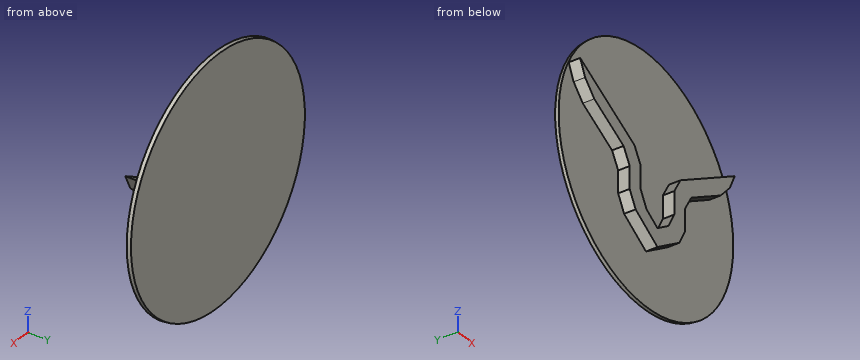
from build123d import *

# Parameters (mm, degrees)
PAD_DEPTH    = 20
SKETCH001_R  = 160.213684
PAD001_DEPTH = 5
PAD001_TAPER = -7
CHAMFER_SIZE = 13


with BuildPart() as part:
    # Sketch → Pad (new body)
    with BuildSketch(Plane.XZ):
        Polygon((0, -88.645294), (51.118267, -54.973317), (51.118267, 0), (127.669846, 44.197075), (142.406095, 75.799063), (31.118267, 11.547005), (31.118267, -44.19839), (0, -64.69622), (-31.118267, -44.19839), (-31.118267, 11.547005), (-142.406095, 75.799063), (-127.669846, 44.197075), (-51.118267, 0), (-51.118267, -54.973317), align=None)
    extrude(amount=PAD_DEPTH)

    # Sketch001 → Pad001 (join)
    with BuildSketch(Plane.XZ):
        with Locations((0, 2.38974)):
            Circle(SKETCH001_R)
    extrude(amount=PAD001_DEPTH, taper=PAD001_TAPER)

    # Chamfer
    chamfer_edges = [part.edges().sort_by_distance(p)[0] for p in [
        (31.118267, -12.5, 11.547005),
        (31.118267, -12.5, -44.19839),
        (-51.118267, -12.5, -54.973317),
        (-51.118267, -12.5, 0),
        (-127.669846, -12.5, 44.197075),
        (-31.118267, -12.5, 11.547005),
        (-31.118267, -12.5, -44.19839),
        (51.118267, -12.5, -54.973317),
        (51.118267, -12.5, 0),
        (127.669846, -12.5, 44.197075),
    ]]
    chamfer(chamfer_edges, length=CHAMFER_SIZE)


solid = part.part
For this review, take the finished solid that the model builds, in its own axes (mm). Round coordinates to 2 decimals unless told otherwise and drop trailing zeros. Write each loop counter-clockwise with the first axis right and the second up, starting at its lowest first coordinate (ties: lowest second). Pieces come first, ordered by that corner, then holes. Notation, with made-up numbers: M 36.25,43.25 L 64.25,43.25 A24 ccw 64.25,72.25 Z; hole C 47.5,76 d10. An arc over 180 degrees is marked long. Write item = value, one per line. Start each with the question number.
(1) We need section A-A (y = -11.5). Give the boundary of the cut face in (x, z), then the cut area to 3 significant figures.
(2) Clearance check with flat-ended pins moving along their axes: pin 1 Ø5 at (x, y) = (44, -4) entering from -Z; pin 2 Ø1.5 at (x, y) = (42.5, -9) entering from -Z; pin 3 Ø5 at (x, y) = (-39.5, -9.5) entering from +Z. State where each tip first meets the part, or that it passes through.
(3) For line 1 along Y through (x, z) = (15, 113.5); line 2 along X through (y, z) = (-12.25, 61); line 3 along X through (y, z) = (-10.75, -41), list the stretches that pass through material, from the lowest coordinate up.
Results found:
q1.outline = M -142.41,75.8 L -133.16,55.98 L -116.41,37.7 L -62.38,6.5 L -51.12,-13 L -51.12,-41.97 L -40.26,-62.12 L 0,-88.65 L 40.26,-62.12 L 51.12,-41.97 L 51.12,-13 L 62.38,6.5 L 116.41,37.7 L 133.16,55.98 L 142.41,75.8 L 42.38,18.05 L 31.12,-1.45 L 31.12,-31.2 L 20.26,-51.35 L 0,-64.7 L -20.26,-51.35 L -31.12,-31.2 L -31.12,-1.45 L -42.38,18.05 Z
q1.area = 8,420 mm²
q2.pin_1 = -152.94
q2.pin_2 = -59.36
q2.pin_3 = 17.39
q3.line_1 = -5 to 0
q3.line_2 = -135.51 to -116.77, 116.77 to 135.51
q3.line_3 = -51.12 to -25.84, 25.84 to 51.12
